Input: dimensioned drawing with shaded views. Units: mm. Origin: part minimum x, y, z. A direction names the side the tool comes from. Coordinates: 2 decimals unless noted, no trailing zeros. Order: outer loops, then holes, each group sorted by start corner. A loop starts at its lowest first (then second) coordinate and runs counter-clockwise, first axis right, second up.
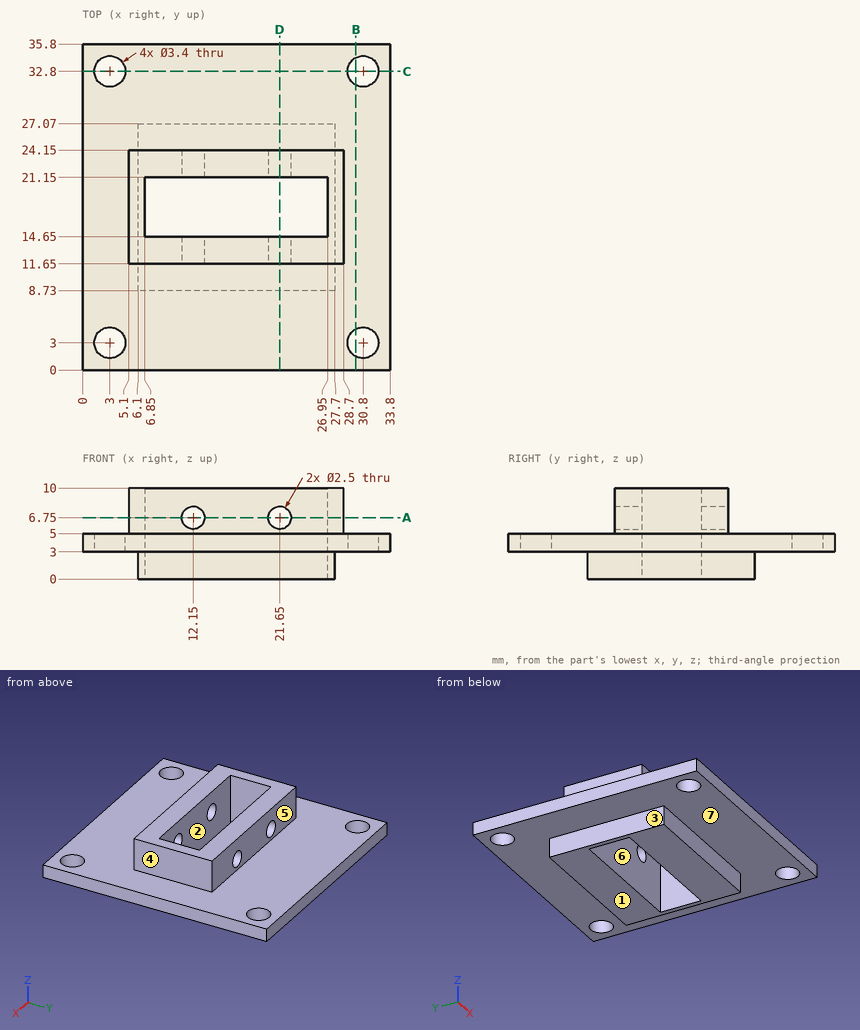
1. Section query C-C, the plane y = 32.8. Output: boundary loops of the cut face in (x, z), plus the area to 3 significant figures.
2. Draft query along Y for the marked faces 5, 6 and 7. Return one class per face: +Y half, -Y half, draft (parallel to the pull), parting line (faces both ways), or undercut.
3. Section query A-A, the plane z = 6.75. Output: boundary loops of the cut face in (x, y).
4. Material intervals for line 1 along Y through (x, z) = (3, 4.5); line 2 along X through (y, z) = (3, 3.7); line 3 along Z through (x, y) = (12.15, 12.6), sorted ascending.
5. Section query D-D, the plane x = 21.65. Output: boundary loops of the cut face in (y, z), plus the area to 3 significant figures.
6. Section query B-B, the plane x = 30. Output: boundary loops of the cut face in (y, z), plus the area to 3 significant figures.
7. Access query for the marked faces 1, 2, 3 and 4. Directions: +Z, -Z, +X, -X, +Y, -Y. A direction counts if a zero-diameter tool reaches every point of the face in a straight line with its end or side. Return the directions, or none.
8. Contact query for flat-ended pins moving along their axis: P1, Ø2, axis at x = 12.15, z = 6.75, coming from the +Y side; P2, Ø5.5, axis at x = 11.5, z = 7.5, coming from the -Y side; P3, Ø5.5, axis at x = 30.8, y = 3, coming from the +Z side; P4, Ø2.5, axis at x = 16.5, z = 1, coming from the -Y side. Output: stop coordinate, or through.
Answer key:
1. outline: (0, 3) - (1.3, 3) - (1.3, 5) - (0, 5) - close; (4.7, 3) - (29.1, 3) - (29.1, 5) - (4.7, 5) - close; (32.5, 3) - (33.8, 3) - (33.8, 5) - (32.5, 5) - close
1. area: 54.0 mm2
2. face 5: +Y half
2. face 6: undercut
2. face 7: draft
3. outline: (5.1, 11.65) - (10.9, 11.65) - (10.9, 14.65) - (6.85, 14.65) - (6.85, 21.15) - (10.9, 21.15) - (10.9, 24.15) - (5.1, 24.15) - close; (13.4, 11.65) - (20.4, 11.65) - (20.4, 14.65) - (13.4, 14.65) - close; (13.4, 21.15) - (20.4, 21.15) - (20.4, 24.15) - (13.4, 24.15) - close; (22.9, 11.65) - (28.7, 11.65) - (28.7, 24.15) - (22.9, 24.15) - (22.9, 21.15) - (26.95, 21.15) - (26.95, 14.65) - (22.9, 14.65) - close
4. line 1: y = 0 to 1.3, 4.7 to 31.1, 34.5 to 35.8
4. line 2: x = 0 to 1.3, 4.7 to 29.1, 32.5 to 33.8
4. line 3: z = 0 to 5.5, 8 to 10
5. outline: (0, 3) - (8.73, 3) - (8.73, 0) - (14.65, 0) - (14.65, 5.5) - (11.65, 5.5) - (11.65, 5) - (0, 5) - close; (11.65, 8) - (14.65, 8) - (14.65, 10) - (11.65, 10) - close; (21.15, 0) - (27.07, 0) - (27.07, 3) - (35.8, 3) - (35.8, 5) - (24.15, 5) - (24.15, 5.5) - (21.15, 5.5) - close; (21.15, 8) - (24.15, 8) - (24.15, 10) - (21.15, 10) - close
5. area: 109 mm2
6. outline: (0, 3) - (1.5, 3) - (1.5, 5) - (0, 5) - close; (4.5, 3) - (31.3, 3) - (31.3, 5) - (4.5, 5) - close; (34.3, 3) - (35.8, 3) - (35.8, 5) - (34.3, 5) - close
6. area: 59.6 mm2
7. face 1: -Z, +X, -X, +Y, -Y
7. face 2: +Z, -Z
7. face 3: -Z, -X, +Y, -Y
7. face 4: +Z, +X, +Y, -Y
8. P1: passes through
8. P2: stops at y = 0
8. P3: stops at z = 5
8. P4: stops at y = 8.73
